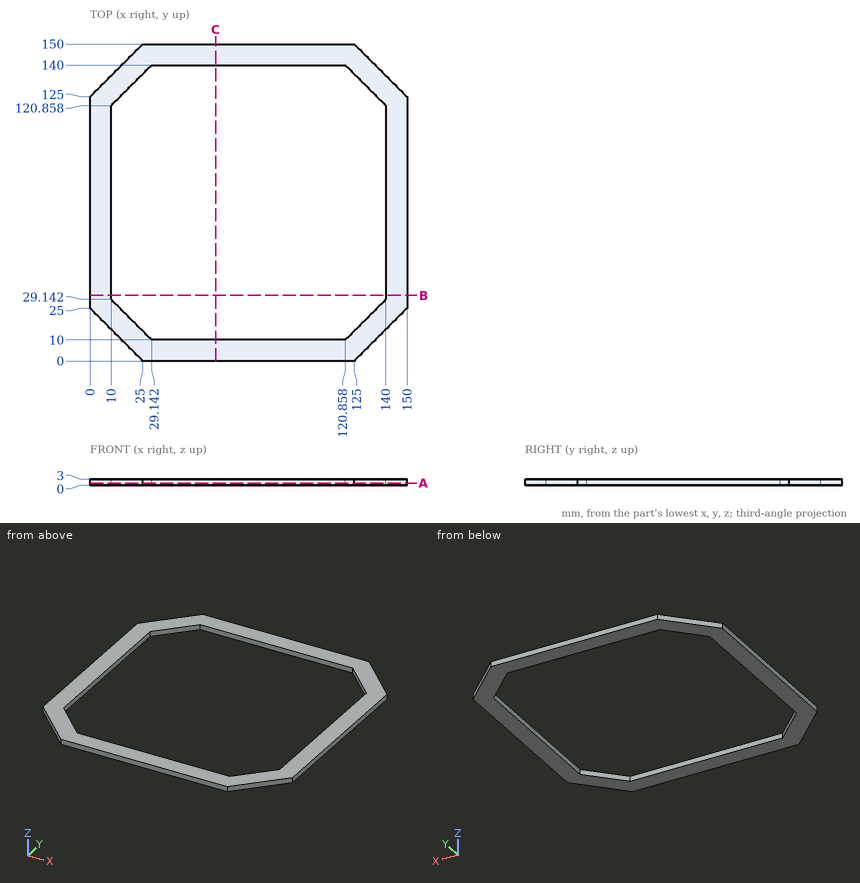
Geometry check sheet. Reference: drawing and pictorial views, mm from the part's lowest x, y, z. Give positions to 0.01 mm unless a question says otherwise; leave off trailing zeros. Write each loop counter-clockwise with the first axis right and the second up, starting at its lowest first coordinate (ties: lowest second). Pieces come first, ordered by that corner, then holes. Notation, with made-up numbers: (-11, 76.5) - (20, 76.5) arc R12 ccw to (20, 94.5) - close; hole circle Ø11 at (12, -13). An arc over 180 degrees is marked (long way). Use a Markdown table: item, result.
Q1. Section check B-B, the plane y = 31. Enter the section's corners in (x, z).
Computed:
| item | result |
|---|---|
| outline | (0, 0) - (10, 0) - (10, 3) - (0, 3) - close; (140, 0) - (150, 0) - (150, 3) - (140, 3) - close |
Q2. Thickness scan on L1, parallel to Y at x = 101.5, z = 0.3; L2, parallel to Y at x = 16, z = 1.95. Record the ranges inside material, lowest first. Write a range as [from, to].
Computed:
| item | result |
|---|---|
| L1 | y = [0, 10], [140, 150] |
| L2 | y = [9, 23.14], [126.86, 141] |
Q3. Section check A-A, the plane z = 1.1. Enter the section's corners in (x, y), then the cut area to 3 significant figures.
Computed:
| item | result |
|---|---|
| outline | (0, 25) - (25, 0) - (125, 0) - (150, 25) - (150, 125) - (125, 150) - (25, 150) - (0, 125) - close; hole (10, 29.14) - (29.14, 10) - (120.86, 10) - (140, 29.14) - (140, 120.86) - (120.86, 140) - (29.14, 140) - (10, 120.86) - close |
| area | 5,080 mm² |
Q4. Go/stop test with a flat-tipped pin: P1, Ø10, axis at x = 128, y = 134.5, coming from the -Z side. Record where the tip stops, or that it passes through.
Computed:
| item | result |
|---|---|
| P1 | stops at z = 0 |
